Check sheet for the modelled part. Datum: model origin and axes. Units: mm. Coordinates: 2 decimals unless noted, no trailing zeros. Loops run counter-clockwise (first coordinate to the right, second up) from the corner with the lowest first, then second, coordinate; pieces in that order, holes last. Notation, with made-up numbers: M 56.25,-39.5 L 81.25,-39.5 A22 cw 81.25,-30.5 Z; hole C 22,29 d6. An arc over 180 degrees is marked long. Return JSON: item names as keys, results as strings.
from build123d import *

# Parameters (mm, degrees)
SKETCH1_R             = 4.5
SKETCH1_R_2           = 4
BOSS_EXTRUDE1_DEPTH   = 10
BOSS_EXTRUDE1_2_DEPTH = 10
BOSS_EXTRUDE4_DEPTH   = 100
BOSS_EXTRUDE5_START   = -10
SKETCH4_R             = 4.5
SKETCH4_R_2           = 4
BOSS_EXTRUDE5_DEPTH   = 10


with BuildPart() as part:
    # Sketch1 → Boss-Extrude1 (new body)
    with BuildSketch(Plane.XY):
        with Locations((-45, 0)):
            Circle(SKETCH1_R)
        with Locations((-45, 0)):
            Circle(SKETCH1_R_2, mode=Mode.SUBTRACT)
    extrude(amount=-BOSS_EXTRUDE1_DEPTH)



with BuildPart() as body_2:
    # Sketch1 → Boss-Extrude1 2 (new body)
    with BuildSketch(Plane.XY):
        with Locations((45, 0)):
            Circle(SKETCH1_R)
        with Locations((45, 0)):
            Circle(SKETCH1_R_2, mode=Mode.SUBTRACT)
    extrude(amount=-BOSS_EXTRUDE1_2_DEPTH)


with BuildPart() as part_1:
    add(part.part)

    add(body_2.part)  # Boss-Extrude4 merges body 2
    # Sketch2 → Boss-Extrude4 (add)
    with BuildSketch(Plane.XY):
        with BuildLine():
            Line((-40.5, 0), (-40.789285714, -0.957242799))
            ThreePointArc((-40.789285714, -0.957242799), (0, -6.986008193), (40.789285714, -0.957242799))
            Line((40.789285714, -0.957242799), (40.5, 0))
            ThreePointArc((40.5, 0), (0, -5.986008193), (-40.5, 0))
        make_face()
    extrude(amount=-BOSS_EXTRUDE4_DEPTH)

    # Sketch4 → Boss-Extrude5 (add)
    # profile 1 of 2: a face of its own
    with BuildSketch(Plane(origin=(0, 0, -100), x_dir=(-1, 0, 0), z_dir=(0, 0, -1)).offset(BOSS_EXTRUDE5_START)):
        with Locations((45, 0)):
            Circle(SKETCH4_R)
        with Locations(Location((45, 0, 0), (0, 0, 180))):
            Circle(SKETCH4_R_2, mode=Mode.SUBTRACT)
    # profile 2 of 2: a face of its own
    with BuildSketch(Plane(origin=(0, 0, -100), x_dir=(-1, 0, 0), z_dir=(0, 0, -1)).offset(BOSS_EXTRUDE5_START)):
        with Locations((-45, 0)):
            Circle(SKETCH4_R)
        with Locations(Location((-45, 0, 0), (0, 0, 180))):
            Circle(SKETCH4_R_2, mode=Mode.SUBTRACT)
    extrude(amount=BOSS_EXTRUDE5_DEPTH)


solid = part_1.part
1) Go/stop test with flat-tipped pins: pin 1 Ø2.5 at (x, y) = (-45, -1) entering from +Z; pin 2 Ø6 at (y, z) = (-1, -47) entering from -X; pin 3 Ø8 at (x, z) = (15, -36.5) entering from +Y; pin 4 Ø10 at (x, z) = (-5, -29) entering from +Y. Record where each tip stops, or that it passes through.
Answers:
{"pin 1": "through", "pin 2": "x = -40.79", "pin 3": "y = -4.69", "pin 4": "y = -5.63"}
2) Section check D-D on x = -18. Record the cut outline in (y, z).
Answers:
{"outline": "M -5.83,-100 L -4.82,-100 L -4.82,0 L -5.83,0 Z"}
3) Section check B-B on y = 1.75. Count the separate pieces of the cut face and the enclosed holes in it, then the cut area to 3 significant figures.
Answers:
{"separate pieces": "8", "enclosed holes": "0", "area": "43.9 mm²"}
4) Section check A-A on x = 45. Record the cut outline in (y, z), then the cut area to 3 significant figures.
Answers:
{"outline": "M -4.5,-100 L -4,-100 L -4,-90 L -4.5,-90 Z; M -4.5,-10 L -4,-10 L -4,0 L -4.5,0 Z; M 4,-100 L 4.5,-100 L 4.5,-90 L 4,-90 Z; M 4,-10 L 4.5,-10 L 4.5,0 L 4,0 Z", "area": "20.0 mm²"}
5) Section check C-C on z = -74. Record the cut outline in (x, y).
Answers:
{"outline": "M -40.79,-0.96 A141 ccw 40.79,-0.96 L 40.5,0 A140 cw -40.5,0 Z"}
6) Scan lines: line 1 along Y through (x, z) = (45, -94); line 2 along Y through (x, z) = (12, -63.5); line 3 along Y through (x, z) = (-32.5, -27). Record each from-to range of solid material in increasing order. Write a range as [from, to].
Answers:
{"line 1": "[-4.5, -4], [4, 4.5]", "line 2": "[-6.47, -5.47]", "line 3": "[-3.19, -2.16]"}
7) Draft check along Y on faces 1 (the face through (41.8, -2.4, -4.9)), 2 (the face through (0.575, -5.985, -49.3)), 3 (the face through (0.2, -6.3, -100)). Enter one of: +Y half, -Y half, draft (parallel to the pull), parting line (faces both ways), or undercut.
Answers:
{"face 1": "undercut", "face 2": "+Y half", "face 3": "draft"}
